Read the model definition and answer for the solid it produces. Units are mm, in the model's axes. Face numbers are marked on the shaded views. Give positions to 0.01 mm unless a question says otherwise; leave off trailing zeros. Loops run counter-clockwise (first coordinate to the right, second up) from the corner with the lowest first, then second, coordinate; pieces in that order, holes last. Notation, with made-up numbers: M -23.75,42.5 L 29.25,42.5 A14 cw 29.25,56.5 Z; hole C -19.75,1.25 d3. An arc over 180 degrees is marked long. Return JSON: item names as keys, results as strings. Group by question number.
```python
from build123d import *

# Parameters (mm, degrees)
SKIZZE1_W                       = 50
SKIZZE1_H                       = 37
AUFSATZ_LINEAR_AUSTRAGEN1_DEPTH = 4
SKIZZE2_W                       = 5.1
SKIZZE2_H                       = 5.1
SCHNITT_LINEAR_AUSTRAGEN1_DEPTH = 37.293175992
SKIZZE3_R                       = 8
SKIZZE3_R_2                     = 5.060953285
AUFSATZ_LINEAR_AUSTRAGEN2_DEPTH = 11
FASE1_SIZE                      = 0.4
SKIZZE4_R                       = 1.265577593
SCHNITT_LINEAR_AUSTRAGEN2_DEPTH = 100


with BuildPart() as part:
    # Skizze1 → Aufsatz-Linear austragen1 (new body)
    with BuildSketch(Plane.XY):
        with Locations((-2.175232088, -5.221327631)):
            Rectangle(SKIZZE1_W, SKIZZE1_H)
    extrude(amount=AUFSATZ_LINEAR_AUSTRAGEN1_DEPTH)

    # Skizze2 → Schnitt-Linear austragen1 (cut, through all)
    with BuildSketch(Plane(origin=(0, 0, 0), x_dir=(-1, 0, 0), z_dir=(0, 0, -1))):
        with Locations((14.725232088, 6.728672369)):
            Rectangle(SKIZZE2_W, SKIZZE2_H)
        with Locations((-12.274767912, 6.728672369)):
            Rectangle(SKIZZE2_W, SKIZZE2_H)
        with Locations((-12.274767912, -17.171327631)):
            Rectangle(SKIZZE2_W, SKIZZE2_H)
        with Locations((14.725232088, -17.171327631)):
            Rectangle(SKIZZE2_W, SKIZZE2_H)
    extrude(amount=-SCHNITT_LINEAR_AUSTRAGEN1_DEPTH, mode=Mode.SUBTRACT)

    # Skizze3 → Aufsatz-Linear austragen2 (add)
    with BuildSketch(Plane(origin=(0, 0, 0), x_dir=(-1, 0, 0), z_dir=(0, 0, -1))):
        with Locations((-9.965334645, -5.221327631)):
            Circle(SKIZZE3_R)
        with Locations((-9.965334645, -5.221327631)):
            Circle(SKIZZE3_R_2, mode=Mode.SUBTRACT)
    extrude(amount=AUFSATZ_LINEAR_AUSTRAGEN2_DEPTH)

    # Fase1
    fase1_edges = [part.edges().sort_by_distance(p)[0] for p in [
        (-2.175232088, 13.278672369, 4),
        (-27.175232088, -5.221327631, 4),
        (-12.175232088, 6.728672369, 4),
        (-12.175232088, 4.178672369, 2),
        (-14.725232088, 9.278672369, 4),
        (-12.175232088, 9.278672369, 2),
        (-17.275232088, 6.728672369, 4),
        (-17.275232088, 9.278672369, 2),
        (-14.725232088, 4.178672369, 4),
        (-17.275232088, 4.178672369, 2),
        (-12.175232088, 6.728672369, 0),
        (-14.725232088, 4.178672369, 0),
        (-17.275232088, 6.728672369, 0),
        (-14.725232088, 9.278672369, 0),
        (14.824767912, -17.171327631, 4),
        (14.824767912, -19.721327631, 2),
        (12.274767912, -14.621327631, 4),
        (14.824767912, -14.621327631, 2),
        (9.724767912, -17.171327631, 4),
        (9.724767912, -14.621327631, 2),
        (12.274767912, -19.721327631, 4),
        (9.724767912, -19.721327631, 2),
        (14.824767912, -17.171327631, 0),
        (12.274767912, -19.721327631, 0),
        (9.724767912, -17.171327631, 0),
        (12.274767912, -14.621327631, 0),
        (-12.175232088, -17.171327631, 4),
        (-12.175232088, -19.721327631, 2),
        (-14.725232088, -14.621327631, 4),
        (-12.175232088, -14.621327631, 2),
        (-17.275232088, -17.171327631, 4),
        (-17.275232088, -14.621327631, 2),
        (-14.725232088, -19.721327631, 4),
        (-17.275232088, -19.721327631, 2),
        (-12.175232088, -17.171327631, 0),
        (-14.725232088, -19.721327631, 0),
        (-17.275232088, -17.171327631, 0),
        (-14.725232088, -14.621327631, 0),
        (14.824767912, 6.728672369, 4),
        (14.824767912, 4.178672369, 2),
        (12.274767912, 9.278672369, 4),
        (-2.175232088, -23.721327631, 4),
        (-27.175232088, -5.221327631, 0),
        (14.824767912, 9.278672369, 2),
        (9.724767912, 6.728672369, 4),
        (9.724767912, 9.278672369, 2),
        (12.274767912, 4.178672369, 4),
        (9.724767912, 4.178672369, 2),
        (14.824767912, 6.728672369, 0),
        (12.274767912, 4.178672369, 0),
        (9.724767912, 6.728672369, 0),
        (12.274767912, 9.278672369, 0),
        (-2.175232088, 13.278672369, 0),
        (22.824767912, -5.221327631, 0),
        (-2.175232088, -23.721327631, 0),
        (15.02628793, -5.221327631, 0),
        (17.965334645, -5.221327631, -11),
        (17.965334645, -5.221327631, 0),
        (-27.175232088, -23.721327631, 2),
        (15.02628793, -5.221327631, -11),
        (-27.175232088, 13.278672369, 2),
        (22.824767912, 13.278672369, 2),
        (22.824767912, -23.721327631, 2),
        (22.824767912, -5.221327631, 4),
    ]]
    chamfer(fase1_edges, length=FASE1_SIZE)

    # Skizze4 → Schnitt-Linear austragen2 (cut, symmetric)
    with BuildSketch(Plane(origin=(0, 0, 0), x_dir=(1, 0, 0), z_dir=(0, 1, 0))):
        with Locations(Location((9.965334645, 4.963129901, 0), (0, 0, 270))):
            Circle(SKIZZE4_R)
    extrude(amount=SCHNITT_LINEAR_AUSTRAGEN2_DEPTH, both=True, mode=Mode.SUBTRACT)


solid = part.part
```
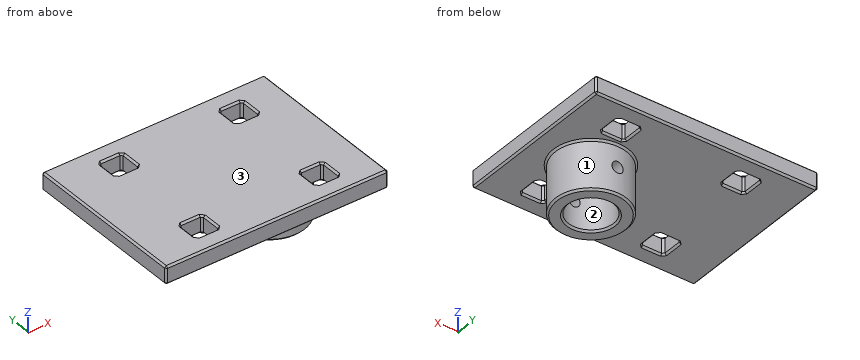
1. Find section B-B (z = -4.5). Write down the section's boundary in (x, y), and give its area (3 significant figures).
2. Find section A-A (y = -18.5). Write down the section's boundary in (x, z), and give its area (3 significant figures).
3. Straight lines are drawn through the part: line 1 along X through (y, z) = (5.5, 1.25); line 2 along Z through (x, y) = (-16, -3); line 3 along X through (y, z) = (-6.5, -3.5). For each, find the intervals that lie inside material, in ascending order.
4. Find section D-D (z = 2). State how many separate pieces and enclosed holes the cut face has, and give its area (3 significant figures).
5. Flat-ended cylindrical pins translate along their axes: P1, Ø3, axis at y = -12.5, z = -9.5, coming from the -X side; P2, Ø6, axis at x = -3.5, y = -14, coming from the -Z side. Find the tip coordinate at first contact, or state that the pin passes through.
6. Find section C-C (x = -23). Write down the section's boundary in (y, z).
7. The mould has two halves that part along Y. Classify the marked faces 1, 2 and 3: +Y half, -Y half, draft (parallel to the pull), parting line (faces both ways), or undercut.
Result:
{
 "1": {"outline": "M 8.79,-13.13 L 8.79,-10.14 A5.06 cw 8.79,-0.3 L 8.79,2.69 A8 ccw Z; M 11.14,-13.13 A8 ccw 11.14,2.69 L 11.14,-0.3 A5.06 cw 11.14,-10.14 Z", "area": "107 mm2"},
 "2": {"outline": "M -27.18,0.4 L -26.78,0 L -17.68,0 L -17.28,0.4 L -17.28,3.6 L -17.68,4 L -26.78,4 L -27.18,3.6 Z; M -12.18,0.4 L -11.78,0 L 9.32,0 L 9.72,0.4 L 9.72,3.6 L 9.32,4 L -11.78,4 L -12.18,3.6 Z; M 14.82,0.4 L 15.22,0 L 22.42,0 L 22.82,0.4 L 22.82,3.6 L 22.42,4 L 15.22,4 L 14.82,3.6 Z", "area": "158 mm2"},
 "3": {"line 1": "x = -27.18 to -17.28, -12.18 to 9.72, 14.82 to 22.82", "line 2": "z = 0 to 4", "line 3": "x = 2.07 to 5.07, 14.86 to 17.86"},
 "4": {"separate pieces": "1", "enclosed holes": "4", "area": "1,750 mm2"},
 "5": {"P1": "stops at x = 4.43", "P2": "stops at z = 0"},
 "6": {"outline": "M -23.72,0.4 L -23.32,0 L 12.88,0 L 13.28,0.4 L 13.28,3.6 L 12.88,4 L -23.32,4 L -23.72,3.6 Z"},
 "7": {"face 1": "parting line", "face 2": "undercut", "face 3": "draft"}
}
